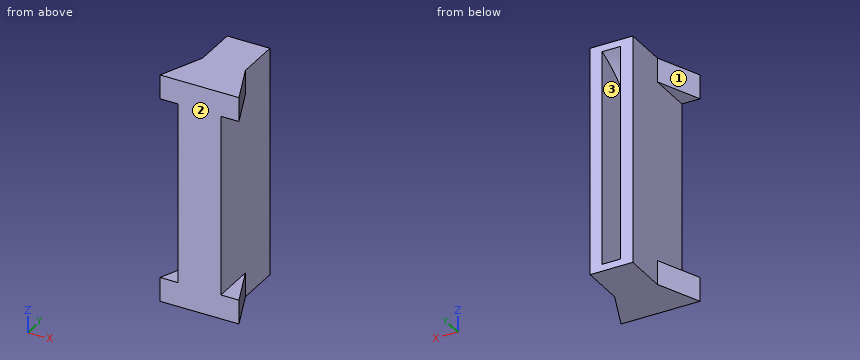
from build123d import *

# Parameters (mm, degrees)
SKETCH1_W                = 35.5
SKETCH1_H                = 190
BOSS_EXTRUDE1_DEPTH      = 72
CUT_EXTRUDE15_DEPTH      = 7.65
CUT_EXTRUDE15_DEPTH_BACK = 7.65
SKETCH2_R                = 95.25
BOSS_EXTRUDE5_DEPTH      = 95
BOSS_EXTRUDE5_DEPTH_BACK = 95
SKETCH7_W                = 41.37003368
SKETCH7_H                = 150
CUT_EXTRUDE16_DEPTH      = 45
SKETCH8_W                = 72.584654809
SKETCH8_H                = 150
CUT_EXTRUDE17_DEPTH      = 45


with BuildPart() as part:
    # Sketch1 → Boss-Extrude1 (new body)
    with BuildSketch(Plane(origin=(0, 0, 0), x_dir=(1, 0, 0), z_dir=(0, 1, 0))):
        Rectangle(SKETCH1_W, SKETCH1_H)
    extrude(amount=BOSS_EXTRUDE1_DEPTH)

    # Sketch2 → Cut-Extrude15 (cut, two sides: drawn at the far end of the back side and taken through both)
    with BuildSketch(Plane(origin=(0, 0, 0), x_dir=(0, 0, -1), z_dir=(1, 0, 0)).offset(-CUT_EXTRUDE15_DEPTH_BACK)):
        with Locations((0, 105.25)):
            Circle(SKETCH2_R)
    extrude(amount=CUT_EXTRUDE15_DEPTH + CUT_EXTRUDE15_DEPTH_BACK, mode=Mode.SUBTRACT)

    # Sketch6 → Boss-Extrude5 (add, two sides: drawn at the far end of the back side and taken through both)
    with BuildSketch(Plane.XY.offset(-BOSS_EXTRUDE5_DEPTH_BACK)):
        Polygon((-17.75, 0), (-32.75, 0), (-17.75, 36), align=None)
        Polygon((17.75, 0), (32.75, 0), (17.75, 36), align=None)
    extrude(amount=BOSS_EXTRUDE5_DEPTH + BOSS_EXTRUDE5_DEPTH_BACK)

    # Sketch7 → Cut-Extrude16 (cut)
    with BuildSketch(Plane(origin=(0, 0, 0), x_dir=(1, 0, 0), z_dir=(0, 1, 0))):
        with Locations((-38.43501684, 0)):
            Rectangle(SKETCH7_W, SKETCH7_H)
    extrude(amount=CUT_EXTRUDE16_DEPTH, mode=Mode.SUBTRACT)

    # Sketch8 → Cut-Extrude17 (cut)
    with BuildSketch(Plane(origin=(0, 0, 0), x_dir=(1, 0, 0), z_dir=(0, 1, 0))):
        with Locations((54.042327404, 0)):
            Rectangle(SKETCH8_W, SKETCH8_H)
    extrude(amount=CUT_EXTRUDE17_DEPTH, mode=Mode.SUBTRACT)


solid = part.part
For this review, take the finished solid that the model builds, in its own axes (mm). Face numbers are marked on the shaded views. Coordinates: 2 decimals unless noted, no trailing zeros. Loops run counter-clockwise (first coordinate to the right, second up) from the corner with the lowest first, then second, coordinate; pieces in that order, holes last. Notation, with made-up numbers: (16, -25) - (30, -25) arc R26 cw to (30, 2) - close; hole circle Ø4 at (-39, 35). An arc over 180 degrees is marked (long way). Return JSON: item names as keys, results as strings.
Item 1: Mouldability with a two-part tool opening along X and no side actions: class the marked faces 1, 2 and 3 as pulls with the +X half, pulls with the -X half, needs draft (parallel to the pull), parting line crosses it, or undercut.
Determined:
{"face 1": "pulls with the -X half", "face 2": "needs draft", "face 3": "undercut"}
Item 2: Take a section at A-A (x = -19.5). Give the boundary of the cut face in (y, z), then the cut area to 3 significant figures.
Determined:
{"outline": "(0, -95) - (31.8, -95) - (31.8, -75) - (0, -75) - close; (0, 75) - (31.8, 75) - (31.8, 95) - (0, 95) - close", "area": "1,270 mm2"}
Item 3: Take a section at B-B (y = 16.5). Give the boundary of the cut face in (x, z) (3 decimals), then the cut area to 3 significant figures.
Determined:
{"outline": "(-25.875, -95) - (25.875, -95) - (25.875, -75) - (17.75, -75) - (17.75, 75) - (25.875, 75) - (25.875, 95) - (-25.875, 95) - (-25.875, 75) - (-17.75, 75) - (-17.75, -75) - (-25.875, -75) - close; hole (-7.65, -34.583) - (7.65, -34.583) - (7.65, 34.583) - (-7.65, 34.583) - close", "area": "6,340 mm2"}
Item 4: Insertion check: pin 1 (21.5 mm diameter, centred on y = 28, z = 44.5, fed in from +X); pin 2 (10 mm diameter, centred on y = 37, z = -28, fed in from -X). Each pin has a flat end and moves straight along its axis. Give the tip position at first contact, or say it passes through.
Determined:
{"pin 1": "stops at x = 17.75", "pin 2": "stops at x = -17.75"}
Item 5: Take a section at C-C (z = 54). Give the boundary of the cut face in (x, y), then the cut area to 3 significant figures.
Determined:
{"outline": "(-17.75, 0) - (17.75, 0) - (17.75, 72) - (7.65, 72) - (7.65, 26.79) - (-7.65, 26.79) - (-7.65, 72) - (-17.75, 72) - close", "area": "1,860 mm2"}
Item 6: Take a section at D-D (y = 28.5). Give the boundary of the cut face in (x, z) (3 decimals).
Determined:
{"outline": "(-20.875, -95) - (20.875, -95) - (20.875, -75) - (17.75, -75) - (17.75, 75) - (20.875, 75) - (20.875, 95) - (-20.875, 95) - (-20.875, 75) - (-17.75, 75) - (-17.75, -75) - (-20.875, -75) - close; hole (-7.65, -56.409) - (7.65, -56.409) - (7.65, 56.409) - (-7.65, 56.409) - close"}
Item 7: For line 1 (X direction, y = 39, z = -37); line 2 (Z direction, x = 18, y = 6.5); line 3 (X direction, y = 8.5, z = 6.5), list the stretches that pass through material, from the lowest coordinate up.
Determined:
{"line 1": "x = -17.75 to -7.65, 7.65 to 17.75", "line 2": "z = -95 to -75, 75 to 95", "line 3": "x = -17.75 to 17.75"}
